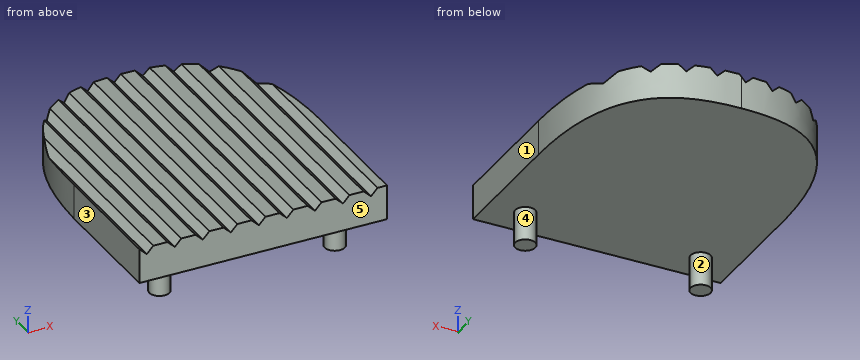
from build123d import *

# Parameters (mm, degrees)
F1_DEPTH = 5.2
F2_R     = 1.5
F3_DEPTH = 5
F5_DEPTH = 47.5


with BuildPart() as f1:
    # F0 (on Top) → F1 (new body)
    with BuildSketch(Plane.XY):
        with BuildLine():
            Line((0.583725, -2.803512), (0.583725, -45.083512))
            Line((0.583725, -45.083512), (19.083725, -45.083512))
            Line((19.083725, -45.083512), (19.083725, -25.983512))
            add(Edge.make_bspline(
                [(0.583725, -2.803512), (9.709766, -2.709429), (19.109245, -5.561374), (19.083725, -25.983512)],
                knots=[29.657417, 29.657417, 29.657417, 29.657417, 59.314835, 59.314835, 59.314835, 59.314835], degree=3))
        make_face()
        with BuildLine():
            Line((-17.916275, -25.983512), (-17.916275, -45.083512))
            Line((-17.916275, -45.083512), (0.583725, -45.083512))
            Line((0.583725, -45.083512), (0.583725, -2.803512))
            add(Edge.make_bspline(
                [(-17.916275, -25.983512), (-17.394919, -5.937705), (-8.542316, -2.897594), (0.583725, -2.803512)],
                knots=[0, 0, 0, 0, 29.657417, 29.657417, 29.657417, 29.657417], degree=3))
        make_face()
    extrude(amount=F1_DEPTH)

    # F2 (on face) → F3 (join)
    with BuildSketch(Plane(origin=(0, 0, 0), x_dir=(1, 0, 0), z_dir=(0, 0, -1))):
        with Locations((-12.516275, 40.383512)):
            Circle(F2_R)
        with Locations((13.683725, 40.383512)):
            Circle(F2_R)
    extrude(amount=F3_DEPTH)

    # F4 (on face) → F5 (cut)
    with BuildSketch(Plane.XZ.offset(45.083512)):
        Polygon((-15.822776, 5.2), (-17.916275, 5.2), (-16.794978, 4.155909), align=None)
        Polygon((-11.635779, 5.2), (-13.729278, 5.2), (-12.607981, 4.155909), align=None)
        Polygon((-7.448782, 5.2), (-9.542281, 5.2), (-8.420984, 4.155909), align=None)
        Polygon((-3.261785, 5.2), (-5.355284, 5.2), (-4.233987, 4.155909), align=None)
        Polygon((0.925212, 5.2), (-1.168287, 5.2), (-0.046989, 4.155909), align=None)
        Polygon((5.112209, 5.2), (3.01871, 5.2), (4.140008, 4.155909), align=None)
        Polygon((8.327005, 4.155909), (9.299206, 5.2), (7.205707, 5.2), align=None)
        Polygon((12.514002, 4.155909), (13.486203, 5.2), (11.392704, 5.2), align=None)
        Polygon((16.700999, 4.155909), (17.6732, 5.2), (15.579701, 5.2), align=None)
    extrude(amount=-F5_DEPTH, mode=Mode.SUBTRACT)


solid = f1.part
Check sheet for the modelled part. Datum: model origin and axes. Units: mm. Face numbers are marked on the shaded views. A direction names the side the tool comes from. Coordinates: 2 decimals unless noted, no trailing zeros. Loops run counter-clockwise (first coordinate to the right, second up) from the corner with the lowest first, then second, coordinate; pieces in that order, holes last. Notation, with made-up numbers: (2, 3.5) -> (52, 3.5) arc R33 cw to (52, 33.5) -> close; hole circle Ø6 at (49.5, 65.25). An arc over 180 degrees is marked (long way). Write item = value, one per line. Start each with the question number.
1. Draft check along X on the marked faces 1, 2 and 3. Enter one of: released by +X, released by -X, zero draft, split by the parting line, or undercut.
2. Section check B-B on z = -4. Record the cut outline in (x, y), then the cut area to 3 significant figures.
3. Depth check by flat-ended pin: P1, Ø4, axis at y = -15.5, z = 3, coming from the -X side; P2, Ø18.5, axis at x = 1, y = -21.5, coming from the -Z side. Enter the tip coordinate at first touch or a pass-through.
4. Material ranges on line 1 (Z direction, x = 14, y = -26); line 2 (Y direction, x = 2, z = 3.75); line 3 (Z direction, x = 11.5, y = -5.5), recorded low to high.
5. Tool access check on the marked faces 4 and 5. Record the directions out of +Z, -Z, +X, -X, +Y, -Y that give a thin tool (end or side, any length) a straight path to the whole face; none if there is none.
Responses:
q1.face_1 = released by +X
q1.face_2 = undercut
q1.face_3 = released by -X
q2.outline = circle Ø3 at (-12.52, -40.38); circle Ø3 at (13.68, -40.38)
q2.area = 14.1 mm2
q3.P1 = -17.04
q3.P2 = 0
q4.line_1 = 0 to 5.2
q4.line_2 = -45.08 to -2.81
q4.line_3 = 0 to 5.1
q5.face_4 = -Z
q5.face_5 = +Z, -Z, +X, -X, -Y
